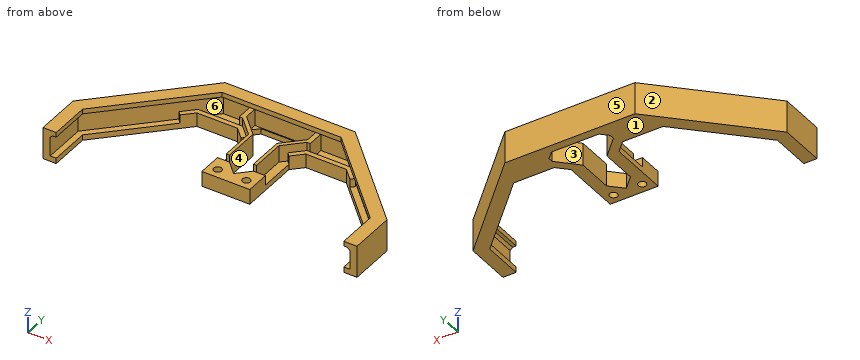
```python
from build123d import *

# Parameters (mm, degrees)
ESBO_O4_R                = 1.65
RESSALTO_EXTRUS_O1_DEPTH = 2.3
RESSALTO_EXTRUS_O2_DEPTH = 3.5
RESSALTO_EXTRUS_O3_DEPTH = 11
CORTE_EXTRUS_O1_DEPTH    = 10.5
CORTE_EXTRUS_O2_DEPTH    = 40.5
RESSALTO_EXTRUS_O4_DEPTH = 2
CHANFRO1_SIZE            = 1
ESBO_O11_R               = 1.65
RESSALTO_EXTRUS_O5_DEPTH = 4
RESSALTO_EXTRUS_O6_DEPTH = 7


with BuildPart() as part:
    # Esboço4 → Ressalto-extrusão1 (new body)
    with BuildSketch(Plane.XY):
        Polygon((70, 0), (70, 28.994949366), (28.994949366, 70), (-28.994949366, 70), (-70, 28.994949366), (-70, 0), (-60, 0), (-60, 24.852813742), (-42.426406871, 42.426406871), (-31.166522241, 53.686291501), (-14.242640687, 53.686291501), (-10, 49.443650814), (-10, 24.443650814), (10, 24.443650814), (10, 49.443650814), (14.242640687, 53.686291501), (31.166522241, 53.686291501), (42.426406871, 42.426406871), (60, 24.852813742), (60, 0), align=None)
        with Locations((6, 28.443650814)):
            Circle(ESBO_O4_R, mode=Mode.SUBTRACT)
        with Locations(Location((-6, 28.443650814, 0), (0, 0, 180))):
            Circle(ESBO_O4_R, mode=Mode.SUBTRACT)
        Polygon((-9.894556364, 62.105443636), (9.894556364, 62.105443636), (12.778174593, 59.221825407), (12.778174593, 57.221825407), (5, 49.443650814), (5, 34.443650814), (0, 29.443650814), (-5, 34.443650814), (-5, 49.443650814), (-12.778174593, 57.221825407), (-12.778174593, 59.221825407), align=None, mode=Mode.SUBTRACT)
    extrude(amount=RESSALTO_EXTRUS_O1_DEPTH)

    # Esboço6 → Ressalto-extrusão2 (add)
    with BuildSketch(Plane.XY.offset(2.3)):
        Polygon((-10, 49.443650814), (-14.242640687, 53.686291501), (-31.166522241, 53.686291501), (-35.409162928, 49.443650814), (-36.823376491, 50.857864376), (-31.994949366, 55.686291501), (-31.166522241, 55.686291501), (-13.414213562, 55.686291501), (-8.585786438, 50.857864376), align=None)
        Polygon((8.585786438, 50.857864376), (13.414213562, 55.686291501), (31.166522241, 55.686291501), (31.994949366, 55.686291501), (36.823376491, 50.857864376), (35.409162928, 49.443650814), (31.166522241, 53.686291501), (14.242640687, 53.686291501), (10, 49.443650814), align=None)
    extrude(amount=RESSALTO_EXTRUS_O2_DEPTH)

    # Esboço7 → Ressalto-extrusão3 (add)
    with BuildSketch(Plane.XY.offset(2.3)):
        Polygon((27.130988335, 65.5), (-27.130988335, 65.5), (-65.5, 27.130988335), (-65.5, 0), (-62.5, 0), (-62.5, 25.888347648), (-25.888347648, 62.5), (25.888347648, 62.5), (62.5, 25.888347648), (62.5, 0), (65.5, 0), (65.5, 27.130988335), align=None)
    extrude(amount=RESSALTO_EXTRUS_O3_DEPTH)

    # Esboço8 → Corte-extrusão1 (cut)
    with BuildSketch(Plane.XY.offset(2.3)):
        Polygon((-65.5, 0), (-65.5, 27.130988335), (-27.130988335, 65.5), (27.130988335, 65.5), (65.5, 27.130988335), (65.5, 0), (65.5, -7.47317723), (91.763905533, -7.47317723), (91.763905533, 81.084833901), (-91.763905533, 81.084833901), (-91.763905533, -7.47317723), (-65.5, -7.47317723), align=None)
    extrude(amount=-CORTE_EXTRUS_O1_DEPTH, mode=Mode.SUBTRACT)

    # Esboço9 → Corte-extrusão2 (cut)
    with BuildSketch(Plane(origin=(0, 0, 0), x_dir=(-1, 0, 0), z_dir=(0, 0, -1))):
        Polygon((60, 0), (70, 0), (70, 8.000623443), (-93.298268705, 8.000623443), (-93.298268705, 0), align=None)
    extrude(amount=-CORTE_EXTRUS_O2_DEPTH, mode=Mode.SUBTRACT)

    # Esboço10 → Ressalto-extrusão4 (add)
    with BuildSketch(Plane.XY.offset(13.3)):
        Polygon((-62.5, 8.000623443), (-62.5, 25.888347648), (-25.888347648, 62.5), (25.888347648, 62.5), (62.5, 25.888347648), (62.5, 8.000623443), (60, 8.000623443), (60, 24.852813742), (24.852813742, 60), (-24.852813742, 60), (-60, 24.852813742), (-60, 8.000623443), align=None)
    extrude(amount=-RESSALTO_EXTRUS_O4_DEPTH)

    # Chanfro1
    chanfro1_edges = [part.edges().sort_by_distance(p)[0] for p in [
        (-62.5, 16.944485546, 11.3),
        (-44.194173824, 44.194173824, 11.3),
        (0, 62.5, 11.3),
        (44.194173824, 44.194173824, 11.3),
        (62.5, 16.944485546, 11.3),
    ]]
    chamfer(chanfro1_edges, length=CHANFRO1_SIZE)

    # Esboço11 → Ressalto-extrusão5 (add)
    with BuildSketch(Plane.XY.offset(2.3)):
        Polygon((-10, 24.443650814), (10, 24.443650814), (10, 34.443650814), (5, 34.443650814), (0, 29.443650814), (-5, 34.443650814), (-10, 34.443650814), align=None)
        with Locations(Location((-6, 28.443650814, 0), (0, 0, 180))):
            Circle(ESBO_O11_R, mode=Mode.SUBTRACT)
        with Locations((6, 28.443650814)):
            Circle(ESBO_O11_R, mode=Mode.SUBTRACT)
    extrude(amount=RESSALTO_EXTRUS_O5_DEPTH)

    # Esboço12 → Ressalto-extrusão6 (add)
    with BuildSketch(Plane.XY.offset(2.3)):
        Polygon((-5, 34.443650814), (-5, 49.443650814), (-12.778174593, 57.221825407), (-12.778174593, 62.936367936), (-14.778174593, 62.936367936), (-14.778174593, 55.686291501), (-13.414213562, 55.686291501), (-6.343145751, 48.615223689), (-6.343145751, 34.443650814), align=None)
        Polygon((6.343145751, 34.443650814), (5, 34.443650814), (5, 49.443650814), (12.778174593, 57.221825407), (12.778174593, 62.936367936), (14.778174593, 62.936367936), (14.778174593, 55.686291501), (13.414213562, 55.686291501), (6.343145751, 48.615223689), align=None)
    extrude(amount=RESSALTO_EXTRUS_O6_DEPTH)


solid = part.part
```
Part model, mm, in its own coordinate system. Face numbers are marked on the shaded views. A direction names the side the tool comes from. Round coordinates to 2 decimals unless told otherwise and drop trailing zeros. Loops run counter-clockwise (first coordinate to the right, second up) from the corner with the lowest first, then second, coordinate; pieces in that order, holes last. Notation, with made-up numbers: (-26.5, 69) -> (18.5, 69) arc R22 ccw to (18.5, 99) -> close; hole circle Ø5 at (-12.75, 1.25). An arc over 180 degrees is marked (long way). Use one line per item in the form item = value. Start each with the question number.
Item 1: Drop flat-ended pins along their axis: pin 1 Ø5 at (x, y) = (-21.5, 53.5) entering from +Z; pin 2 Ø1.1 at (x, y) = (9, 39.5) entering from +Z; pin 3 Ø0.7 at (x, z) = (-14, 8) entering from -Y. Give the stop position or say it passes through.
Item 2: Tool access for the marked faces 4, 5 and 6: list every direction of +Z, -Z, +X, -X, +Y, -Y with a clear straight run to the whole face (end or side of a thin tool).
Item 3: Band-saw the part on A-A (y = 16). List the corners of the cut face in (x, z), plus the area to 3 significant figures.
Item 4: Two-plate mould, pull along Y, no slides. Class the marked faces 1, 2 and 3: released by +Y, released by -Y, zero draft, split by the parting line, or undercut.
Item 5: Drill centre lines: line 1 along X through (y, z) = (16, 9.75); line 2 along Z through (x, y) = (60.5, 24); line 3 along X through (y, z) = (56.5, 3.5). Where is each one in solid material? Low to high.
Data:
q1.pin_1 = 5.8
q1.pin_2 = 2.3
q1.pin_3 = 55.69
q2.face_4 = +Z, -Z
q2.face_5 = +Z, -Z, +X, -X, +Y
q2.face_6 = none
q3.outline = (-65.5, 0) -> (-60, 0) -> (-60, 2.3) -> (-62.5, 2.3) -> (-62.5, 10.3) -> (-61.5, 11.3) -> (-60, 11.3) -> (-60, 13.3) -> (-65.5, 13.3) -> close; (60, 0) -> (65.5, 0) -> (65.5, 13.3) -> (60, 13.3) -> (60, 11.3) -> (61.5, 11.3) -> (62.5, 10.3) -> (62.5, 2.3) -> (60, 2.3) -> close
q3.area = 102 mm^2
q4.face_1 = zero draft
q4.face_2 = released by +Y
q4.face_3 = undercut
q5.line_1 = -65.5 to -62.5, 62.5 to 65.5
q5.line_2 = 0 to 2.3, 11.3 to 13.3
q5.line_3 = -36.13 to -31.89, -14.78 to -12.06, 12.06 to 14.78, 31.89 to 36.13
